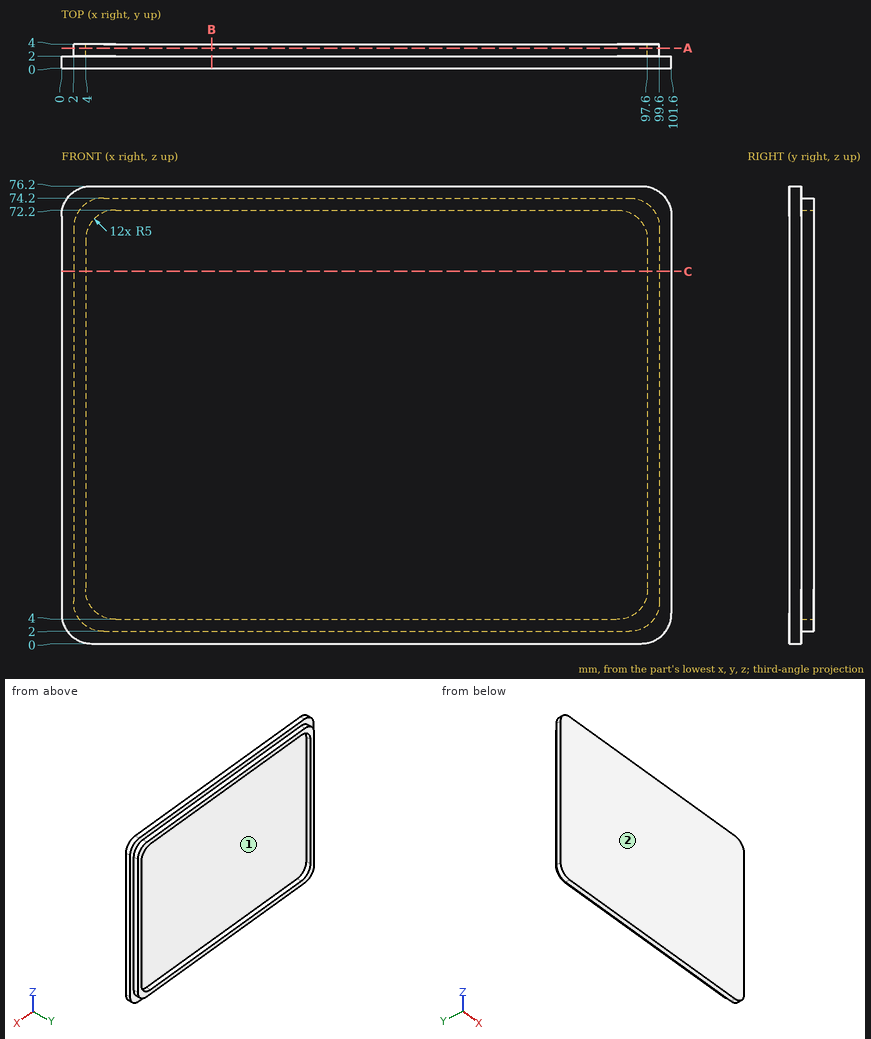
The drawing under review shows one solid part. Ordinate dimensions are in mm from its lowest x, y, z. Give positions to 0.01 mm unless a question says otherwise; leave off trailing zeros. Order: outer loops, then holes, each group sorted by start corner. A loop starts at its lowest first (then second) coordinate and runs counter-clockwise, first axis right, second up. Notation, with made-up numbers: (48.25, -32.5) -> (104.25, -32.5) arc R33 cw to (104.25, 2.5) -> close; hole circle Ø8 at (-38, -27.5). An arc over 180 degrees is marked (long way). Write item = value, one per line.
1) We need section B-B, the plane x = 25. Give the boundary of the cut face in (y, z).
Findings:
outline = (0, 0) -> (2, 0) -> (2, 2) -> (4, 2) -> (4, 4) -> (2, 4) -> (2, 72.2) -> (4, 72.2) -> (4, 74.2) -> (2, 74.2) -> (2, 76.2) -> (0, 76.2) -> close
2) We need section C-C, the plane z = 62. Give the boundary of the cut face in (x, y), and give its area (3 significant figures).
Findings:
outline = (0, 0) -> (101.6, 0) -> (101.6, 2) -> (99.6, 2) -> (99.6, 4) -> (97.6, 4) -> (97.6, 2) -> (4, 2) -> (4, 4) -> (2, 4) -> (2, 2) -> (0, 2) -> close
area = 211 mm^2
3) Draft analysis for pull direction X (two halves, no side actions). For the marked faces 1 and 2, state which applies: pulls with the +X half, pulls with the -X half, needs draft (parallel to the pull), parting line crosses it, or undercut.
Findings:
face_1 = undercut
face_2 = needs draft
4) To check wall thickness, follow L1, parallel to X at y = 2.8, z = 64.5; L2, parallel to Z at x = 81.5, y = 2.1; L3, parallel to Y at x = 29, z = 55.5. State the ranges of each line that lie inside material, in increasing order. Write a range as from..to.
Findings:
L1 = 2..4, 97.6..99.6
L2 = 2..4, 72.2..74.2
L3 = 0..2
5) We need section A-A, the plane y = 3.3. Give the boundary of the cut face in (x, z), and give its area (3 significant figures).
Findings:
outline = (2, 7) arc R5 ccw to (7, 2) -> (94.6, 2) arc R5 ccw to (99.6, 7) -> (99.6, 69.2) arc R5 ccw to (94.6, 74.2) -> (7, 74.2) arc R5 ccw to (2, 69.2) -> close; hole (4, 9) arc R5 ccw to (9, 4) -> (92.6, 4) arc R5 ccw to (97.6, 9) -> (97.6, 67.2) arc R5 ccw to (92.6, 72.2) -> (9, 72.2) arc R5 ccw to (4, 67.2) -> close
area = 663 mm^2
6) Insertion check: pin 1 (0.6 mm diameter, centred on y = 2.5, z = 35, fed in from +X); pin 2 (1.6 mm diameter, centred on y = 3.5, z = 27.5, fed in from -X); pin 3 (1 mm diameter, centred on x = 51, y = 3, fed in from +Z). Each pin has a flat end and moves straight along its axis. Give the tip position at first contact, or say it passes through.
Findings:
pin_1 = 99.6
pin_2 = 2
pin_3 = 74.2
